from build123d import *

# Parameters (mm, degrees)
SKETCH1_W            = 50.8
SKETCH1_H            = 50.8
BOSS_EXTRUDE1_DEPTH  = 2.54
SKETCH2_R            = 19.05
CUT_EXTRUDE1_DEPTH   = 37.010715072
SKETCH3_R            = 1.905
CUT_EXTRUDE2_DEPTH   = 37.010715072
SKETCH4_W            = 21.59
SKETCH4_H            = 9.70380699
CUT_EXTRUDE3_DEPTH   = 37.010715072
SKETCH5_W            = 3.175
SKETCH5_H            = 19.05
BOSS_EXTRUDE2_DEPTH  = 35.005772
SKETCH6_W            = 50.8
SKETCH6_H            = 50.8
BOSS_EXTRUDE3_DEPTH  = 2.54
SKETCH8_W            = 50.8
SKETCH8_H            = 37.545772
BOSS_EXTRUDE4_DEPTH  = 2.54
SKETCH9_R            = 3.048
BOSS_EXTRUDE5_DEPTH  = 5.08
CUT_EXTRUDE4_REACH   = 53.962
SKETCH10_W           = 22.86
SKETCH10_H           = 10.16
SKETCH13_W           = 50.8
SKETCH13_H           = 2.54
BOSS_EXTRUDE7_DEPTH  = 57.15
SKETCH15_W           = 3.175
SKETCH15_H           = 12.7
BOSS_EXTRUDE8_DEPTH  = 25.4
SKETCH17_W           = 3.175
SKETCH17_H           = 12.7
BOSS_EXTRUDE10_DEPTH = 25.4
SKETCH18_W           = 3.175
SKETCH18_H           = 32.465772
BOSS_EXTRUDE11_DEPTH = 25.4


with BuildPart() as part:
    # Sketch1 → Boss-Extrude1 (new body)
    with BuildSketch(Plane(origin=(0, 0, 0), x_dir=(1, 0, 0), z_dir=(0, 1, 0))):
        Rectangle(SKETCH1_W, SKETCH1_H)
    extrude(amount=BOSS_EXTRUDE1_DEPTH)

    # Sketch2 → Cut-Extrude1 (cut, through all)
    with BuildSketch(Plane(origin=(0, 2.54, 0), x_dir=(1, 0, 0), z_dir=(0, 1, 0))):
        with Locations(Location((0, 0, 0), (0, 0, 270))):
            Circle(SKETCH2_R)
    extrude(amount=-CUT_EXTRUDE1_DEPTH, mode=Mode.SUBTRACT)

    # Sketch3 → Cut-Extrude2 (cut, through all)
    with BuildSketch(Plane(origin=(0, 2.54, 0), x_dir=(1, 0, 0), z_dir=(0, 1, 0))):
        with Locations(Location((-15.494, 15.494, 0), (0, 0, 270))):
            Circle(SKETCH3_R)
        with Locations(Location((15.494, 15.494, 0), (0, 0, 270))):
            Circle(SKETCH3_R)
        with Locations(Location((15.494, -15.494, 0), (0, 0, 270))):
            Circle(SKETCH3_R)
        with Locations(Location((-15.494, -15.494, 0), (0, 0, 270))):
            Circle(SKETCH3_R)
    extrude(amount=-CUT_EXTRUDE2_DEPTH, mode=Mode.SUBTRACT)

    # Sketch4 → Cut-Extrude3 (cut, through all)
    with BuildSketch(Plane(origin=(0, 2.54, 0), x_dir=(1, 0, 0), z_dir=(0, 1, 0))):
        with Locations((0, -20.548096505)):
            Rectangle(SKETCH4_W, SKETCH4_H)
    extrude(amount=-CUT_EXTRUDE3_DEPTH, mode=Mode.SUBTRACT)

    # Sketch5 → Boss-Extrude2 (add)
    with BuildSketch(Plane(origin=(0, 2.54, 0), x_dir=(1, 0, 0), z_dir=(0, 1, 0))):
        with Locations((-23.8125, -15.875)):
            Rectangle(SKETCH5_W, SKETCH5_H)
        with Locations((23.8125, -15.875)):
            Rectangle(SKETCH5_W, SKETCH5_H)
    extrude(amount=BOSS_EXTRUDE2_DEPTH)

    # Sketch6 → Boss-Extrude3 (add)
    with BuildSketch(Plane(origin=(0, 37.545772, 0), x_dir=(1, 0, 0), z_dir=(0, 1, 0))):
        Rectangle(SKETCH6_W, SKETCH6_H)
    extrude(amount=-BOSS_EXTRUDE3_DEPTH)

    # Sketch8 → Boss-Extrude4 (add)
    with BuildSketch(Plane.XY.offset(25.4)):
        with Locations((0, 18.772886)):
            Rectangle(SKETCH8_W, SKETCH8_H)
    extrude(amount=-BOSS_EXTRUDE4_DEPTH)

    # Sketch9 → Boss-Extrude5 (add)
    with BuildSketch(Plane.XZ.offset(-35.005772)):
        with Locations(Location((0, 0, 0), (0, 0, 270))):
            Circle(SKETCH9_R)
    extrude(amount=BOSS_EXTRUDE5_DEPTH)

    # Sketch10 → Cut-Extrude4 (cut, up to next)
    with BuildSketch(Plane.XZ, mode=Mode.PRIVATE) as cut_extrude4_sk1:
        with Locations((0, -20.32)):
            Rectangle(SKETCH10_W, SKETCH10_H)
    cut_extrude4_tool1 = extrude(cut_extrude4_sk1.sketch, amount=-CUT_EXTRUDE4_REACH, mode=Mode.PRIVATE) & part.part
    add(cut_extrude4_tool1.solids().sort_by_distance((0, 0, -20.32))[0], mode=Mode.SUBTRACT)

    # Sketch13 → Boss-Extrude7 (add)
    with BuildSketch(Plane(origin=(25.4, 0, 0), x_dir=(0, 0, -1), z_dir=(1, 0, 0))):
        with Locations((0, 36.275772)):
            Rectangle(SKETCH13_W, SKETCH13_H)
        with Locations((0, 1.27)):
            Rectangle(SKETCH13_W, SKETCH13_H)
    extrude(amount=BOSS_EXTRUDE7_DEPTH)

    # Sketch15 → Boss-Extrude8 (add)
    with BuildSketch(Plane(origin=(0, 37.545772, 0), x_dir=(1, 0, 0), z_dir=(0, 1, 0))):
        with Locations((80.9625, 19.05)):
            Rectangle(SKETCH15_W, SKETCH15_H)
        with Locations((80.9625, -19.05)):
            Rectangle(SKETCH15_W, SKETCH15_H)
    extrude(amount=BOSS_EXTRUDE8_DEPTH)

    # Sketch17 → Boss-Extrude10 (add)
    with BuildSketch(Plane(origin=(0, 2.54, 0), x_dir=(1, 0, 0), z_dir=(0, 1, 0))):
        with Locations((80.9625, -19.05)):
            Rectangle(SKETCH17_W, SKETCH17_H)
        with Locations((80.9625, 19.05)):
            Rectangle(SKETCH17_W, SKETCH17_H)
    extrude(amount=BOSS_EXTRUDE10_DEPTH)

    # Sketch18 → Boss-Extrude11 (add)
    with BuildSketch(Plane(origin=(25.4, 0, 0), x_dir=(0, 0, -1), z_dir=(1, 0, 0))):
        with Locations((-14.2875, 18.772886)):
            Rectangle(SKETCH18_W, SKETCH18_H)
    extrude(amount=BOSS_EXTRUDE11_DEPTH)


solid = part.part
Geometry check sheet. Reference: the model listing, model coordinates, mm. A direction names the side the tool comes from. Round coordinates to 2 decimals unless told otherwise and drop trailing zeros. Write each loop counter-clockwise with the first axis right and the second up, starting at its lowest first coordinate (ties: lowest second). Pieces come first, ordered by that corner, then holes. Notation, with made-up numbers: (-16, 48) -> (28, 48) arc R24 ccw to (28, 69) -> close; hole circle Ø10 at (65, 47). An arc over 180 degrees is marked (long way). One line per item, written item: value. Start each with the question number.
(1) Go/stop test with flat-tipped pins: pin 1 Ø5 at (x, z) = (51, 6) entering from +Y; pin 2 Ø17.5 at (x, y) = (7.5, 9) entering from -Z; pin 3 Ø6 at (y, z) = (8.5, 5) entering from +X; pin 4 Ø10 at (x, z) = (0, 16) entering from -Y. Record where each tip stops, or that it passes through.
(2) Scan lines: line 1 (X direction, y = 24.5, z = 21.5) (3 decimals); line 2 (Y direction, x = -19.5, z = 13); line 3 (X direction, y = 56.5, z = -21) (3 decimals). Record each from-to range of solid material in increasing order. Write a range as [from, to].
(3) Cross-section at B-B, the plane y = 16.5. Record the cut outline in (x, z) (3 decimals), and give its area (3 significant figures).
(4) Cross-section at A-A, the plane x = 62. Record the cut outline in (y, z), and give its area (3 significant figures).
(5) Access from +Z, -Z, +X, -X, +Y, -Y to the whole of each face (thin tool, end or side, straight path). Record for faces 4 (the flat face through (38, 19, 15.875)), 5 (the cylindrical face through (2.57, 32.5, -1.64)), 6 (the flat face through (50.8, 19, 14)), 7 (the flat face through (81, 15, -12.7)), 8 (the flat face through (11.43, 1, -20)).
(6) Draft check along Y on faces 1 (the flat face through (81, 62.946, 19)), 2 (the flat face through (79.375, 50, 19)), 3 (the flat face through (25.4, 19, 10)). Enter one of: +Y half, -Y half, draft (parallel to the pull), parting line (faces both ways), or undercut.
(7) Cross-section at D-D, the plane z = 0. Record the cut outline in (x, y).
(8) Cross-section at C-C, the plane y = 33. Record the cut outline in (x, z) (3 decimals).
Answer:
1. pin 1: y = 37.55
1. pin 2: z = -25.4
1. pin 3: x = 25.4
1. pin 4: y = 35.01
2. line 1: [-25.4, -22.225], [22.225, 25.4], [79.375, 82.55]
2. line 2: [0, 2.54], [35.01, 37.55]
2. line 3: [79.375, 82.55]
3. outline: (-25.4, 6.35) -> (-22.225, 6.35) -> (-22.225, 22.86) -> (22.225, 22.86) -> (22.225, 6.35) -> (25.4, 6.35) -> (25.4, 12.7) -> (50.8, 12.7) -> (50.8, 15.875) -> (25.4, 15.875) -> (25.4, 25.4) -> (-25.4, 25.4) -> close; (79.375, -25.4) -> (82.55, -25.4) -> (82.55, -12.7) -> (79.375, -12.7) -> close; (79.375, 12.7) -> (82.55, 12.7) -> (82.55, 25.4) -> (79.375, 25.4) -> close
3. area: 395 mm²
4. outline: (0, -25.4) -> (2.54, -25.4) -> (2.54, 25.4) -> (0, 25.4) -> close; (35.01, -25.4) -> (37.55, -25.4) -> (37.55, 25.4) -> (35.01, 25.4) -> close
4. area: 258 mm²
5. face 4: +Z
5. face 5: -Y
5. face 6: +Z, -Z
5. face 7: +X, -X
5. face 8: -Z, -Y
6. face 1: +Y half
6. face 2: draft
6. face 3: undercut
7. outline: (-25.4, 0) -> (-19.05, 0) -> (-19.05, 2.54) -> (-25.4, 2.54) -> close; (-25.4, 35.01) -> (-3.05, 35.01) -> (-3.05, 29.93) -> (3.05, 29.93) -> (3.05, 35.01) -> (82.55, 35.01) -> (82.55, 37.55) -> (-25.4, 37.55) -> close; (19.05, 0) -> (82.55, 0) -> (82.55, 2.54) -> (19.05, 2.54) -> close
8. outline: (-25.4, 6.35) -> (-22.225, 6.35) -> (-22.225, 22.86) -> (22.225, 22.86) -> (22.225, 6.35) -> (25.4, 6.35) -> (25.4, 12.7) -> (50.8, 12.7) -> (50.8, 15.875) -> (25.4, 15.875) -> (25.4, 25.4) -> (-25.4, 25.4) -> close; circle Ø6.096 at (0, 0)
